Answer from the drawing. Dimensions are ordinates in mm from the lowest x, y and z of the part. A direction names the side the tool comes from. Coordinates: 2 decimals unless noted, no trailing zeros. Write each loop counter-clockwise with the first axis right and the second up, starting at its lowest first coordinate (ties: lowest second). Pieces come first, ordered by that corner, then holes. Notation, with made-up numbers: (14.25, -31) - (49.25, -31) arc R16 cw to (49.25, -15) - close; hole circle Ø2 at (18.5, -26). An arc over 180 degrees is marked (long way). Return JSON: item names as keys, results as strings.
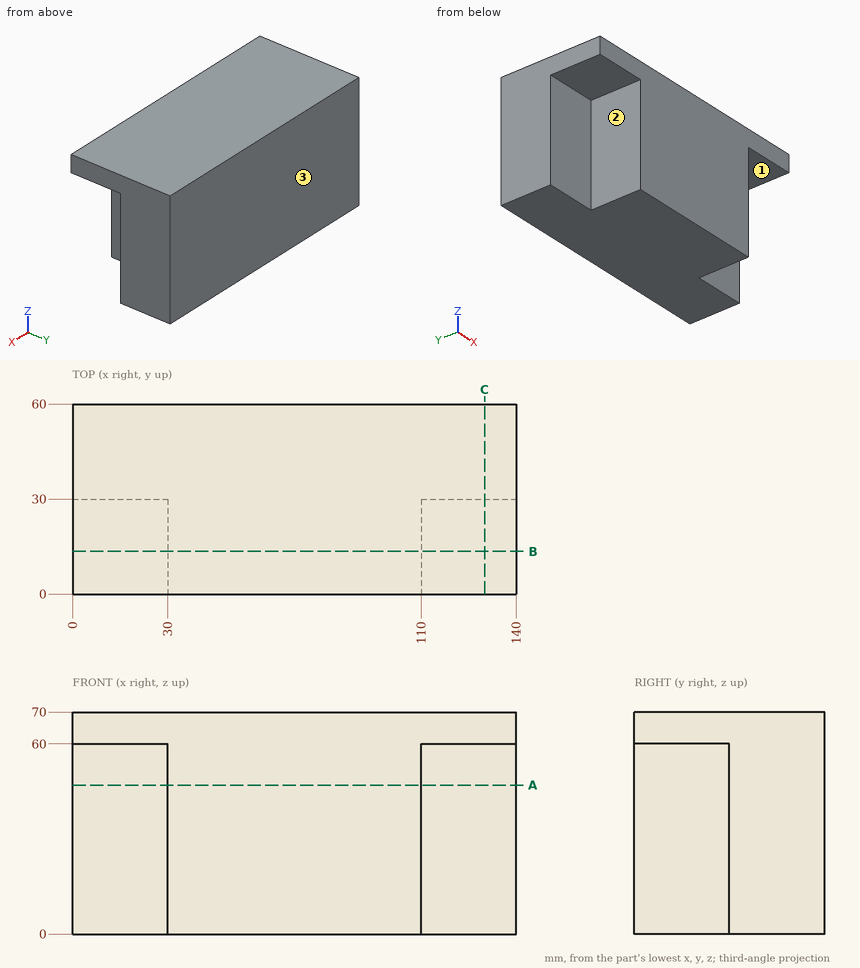
(1) Straight lines are drawn through the part: line 1 (X direction, y = 25, z = 22); line 2 (Y direction, x = 127, z = 23.5); line 3 (Z direction, x = 29, y = 28.5). For each, find the intervals that lie inside material, in ascending order. Write a range as from..to.
Answer:
{"line 1": "30..110", "line 2": "30..60", "line 3": "60..70"}
(2) A cutting plane is placed at A-A (z = 47). Determine the outline of the cut face in (x, y).
Answer:
{"outline": "(0, 30) - (30, 30) - (30, 0) - (110, 0) - (110, 30) - (140, 30) - (140, 60) - (0, 60) - close"}
(3) Which of the six approach directions +Z, -Z, +X, -X, +Y, -Y give full straight-line access (tool end or side, diameter ignored) to the marked faces 1, 2 and 3?
Answer:
{"face 1": "-Z, +X, -Y", "face 2": "-Z, -X, -Y", "face 3": "+Z, -Z, +X, -X, +Y"}
(4) A cutting plane is placed at C-C (x = 130). Determine the outline of the cut face in (y, z).
Answer:
{"outline": "(0, 60) - (30, 60) - (30, 0) - (60, 0) - (60, 70) - (0, 70) - close"}
(5) A cutting plane is placed at B-B (y = 13.5). Determine the outline of the cut face in (x, z).
Answer:
{"outline": "(0, 60) - (30, 60) - (30, 0) - (110, 0) - (110, 60) - (140, 60) - (140, 70) - (0, 70) - close"}
(6) Flat-ended cylindrical pins translate along their axes: P1, Ø9, axis at x = 124, z = 42.5, coming from the -Y side; P2, Ø9, axis at x = 17.5, y = 16.5, coming from the -Z side; P3, Ø15, axis at y = 21, z = 45, coming from the -X side. Find the tip coordinate at first contact, or state that the pin passes through.
Answer:
{"P1": "y = 30", "P2": "z = 60", "P3": "x = 30"}
